from build123d import *

# Parameters (mm, degrees)
F0_R     = 14.95
F1_DEPTH = 15
F2_R     = 7
F3_DEPTH = 15
F4_R     = 0.8
F5_DEPTH = 15


with BuildPart() as f1:
    # F0 (on Top) → F1 (new body)
    with BuildSketch(Plane.XY):
        Circle(F0_R)
    extrude(amount=F1_DEPTH)

    # F2 (on Top) → F3 (cut)
    with BuildSketch(Plane.XY):
        Circle(F2_R)
    extrude(amount=F3_DEPTH, mode=Mode.SUBTRACT)

    # F4 (on Top) → F5 (cut)
    with BuildSketch(Plane.XY):
        with Locations((-11, 0)):
            Circle(F4_R)
        with Locations((11, 0)):
            Circle(F4_R)
    extrude(amount=F5_DEPTH, mode=Mode.SUBTRACT)


solid = f1.part
For this review, take the finished solid that the model builds, in its own axes (mm). Round coordinates to 2 decimals unless told otherwise and drop trailing zeros. Write each loop counter-clockwise with the first axis right and the second up, starting at its lowest first coordinate (ties: lowest second). Pieces come first, ordered by that corner, then holes. Notation, with made-up numbers: M 88.25,46.25 L 131.25,46.25 A7 ccw 131.25,50.25 Z; hole C 78.25,14.5 d3. An arc over 180 degrees is marked long. Write item = value, one per line. Start each with the question number.
(1) For line 1 along Y through (x, z) = (0, 3.75); line 2 along X through (y, z) = (-0.5, 1); line 3 along Y through (x, z) = (-4.5, 7), list the stretches that pass through material, from the lowest coordinate up.
(2) The part is to be moulded in two halves that separate along Y. For faces 1 (the face through (11.763, 0.24, 7.395)), 2 (the face through (-10.237, 0.24, 7.395)), 3 (the face through (6.44, -3.11, 15)), 4 (the face through (6.899, -13.263, 7.395)), say which applies: +Y half, -Y half, draft (parallel to the pull), parting line (faces both ways), or undercut.
(3) We need section D-D (z = 4.75). Give the boundary of the cut face in (x, y), then the cut area to 3 significant figures.
(4) We need section A-A (x = 0). Give the boundary of the cut face in (y, z), then the cut area to 4 significant figures.
(5) We need section B-B (y = 0). Give the boundary of the cut face in (x, z).
(6) We need section C-C (y = 6). Give the boundary of the cut face in (x, z).
(7) Clearance check with flat-ended pins moving along their axes: pin 1 Ø6 at (x, z) = (-7, 6) entering from -Y; pin 2 Ø1.5 at (y, z) = (1, 13) entering from +X; pin 3 Ø1.3 at (x, y) = (-11, 0) entering from -Z; pin 4 Ø4 at (x, y) = (8.5, 9) entering from -Z. State where each tip first meets the part, or that it passes through.
Results found:
q1.line_1 = -14.95 to -7, 7 to 14.95
q1.line_2 = -14.94 to -11.62, -10.38 to -6.98, 6.98 to 10.38, 11.62 to 14.94
q1.line_3 = -14.26 to -5.36, 5.36 to 14.26
q2.face_1 = undercut
q2.face_2 = undercut
q2.face_3 = draft
q2.face_4 = parting line
q3.outline = C 0,0 d29.9; hole C -11,0 d1.6; hole C 0,0 d14; hole C 11,0 d1.6
q3.area = 544 mm²
q4.outline = M -14.95,0 L -7,0 L -7,15 L -14.95,15 Z; M 7,0 L 14.95,0 L 14.95,15 L 7,15 Z
q4.area = 238.5 mm²
q5.outline = M -14.95,0 L -11.8,0 L -11.8,15 L -14.95,15 Z; M -10.2,0 L -7,0 L -7,15 L -10.2,15 Z; M 7,0 L 10.2,0 L 10.2,15 L 7,15 Z; M 11.8,0 L 14.95,0 L 14.95,15 L 11.8,15 Z
q6.outline = M -13.69,0 L -3.61,0 L -3.61,15 L -13.69,15 Z; M 3.61,0 L 13.69,0 L 13.69,15 L 3.61,15 Z
q7.pin_1 = -14.4
q7.pin_2 = 14.95
q7.pin_3 = through
q7.pin_4 = 0
